For this review, take the finished solid that the model builds, in its own axes (mm). A direction names the side the tool comes from. Give positions to 0.01 mm unless a question says otherwise; leave off trailing zeros. Write each loop counter-clockwise with the first axis right and the second up, starting at its lowest first coordinate (ties: lowest second). Pieces come first, ordered by that corner, then holes.
Q1. For line 1 (Y direction, x = -1.5, z = 1.25); line 2 (Y direction, x = -20, z = 5); line 3 (Z direction, x = 0, y = 65.5) (1 decimal), list the stretches that pass through material, from the lowest coordinate up.
Q2. Insertion check: P1, Ø1, axis at x = 33.5, z = 5.5, coming from the +Y side; P2, Ø8, axis at x = -39.2, y = 39.2, coming from the +Z side; P3, Ø8, axis at x = 26, z = 13.5, coming from the -Y side. Each pin has a flat end and moves straight along its axis. Give the tip position at first contact, or say it passes through.
Q3. Mouldability with a two-part tool opening along X and no side actions: class faces 1 (the cylindrical face through (39.531, -36.668, 3.219)), 2 (the cylindrical face through (-14.77, -66.515, 6.574)), 3 (the flat face through (30, -55, 15.875)) as released by +X, released by -X, zero draft, split by the parting line, or undercut.
Q4. Machinability: for faces 4 (the cylindrical face through (36.668, 39.531, 3.219)), 5 (the flat face through (-28, -41, 6.35)), which of the approach directions +Z, -Z, +X, -X, +Y, -Y give a long, thin tool a straight path to every point of the face, cutting with its end or side? Answer none if there is none.
Q5. We need section A-A (z = 2). Write out the cut boundary in (x, y), then the cut area to 3 significant figures.
```python
from build123d import *

# Parameters (mm, degrees)
SKETCH1_R                      = 68.1355
SKETCH1_R_2                    = 49.0855
EXTRUDE1_DEPTH                 = 15.875
SKETCH2_R                      = 61.7855
EXTRUDE2_DEPTH                 = 9.525
TAP_DRILL_FOR_10_32_TAP1_D     = 4.0386
TAP_DRILL_FOR_10_32_TAP1_DEPTH = 12.7
TAP_DRILL_FOR_10_32_TAP1_TIP   = 1.213317848
CIRPATTERN1_COUNT              = 4
CIRPATTERN2_COUNT              = 4
CHAMFER1_SIZE                  = 2.54
CHAMFER1_SIZE2                 = 0.680590949


with BuildPart() as part:
    # Sketch1 → Extrude1 (new body)
    with BuildSketch(Plane.XY):
        Circle(SKETCH1_R)
        Circle(SKETCH1_R_2, mode=Mode.SUBTRACT)
    extrude(amount=EXTRUDE1_DEPTH)

    # Sketch2 → Extrude2 (cut)
    with BuildSketch(Plane.XY.offset(15.875)):
        Circle(SKETCH2_R)
    extrude(amount=-EXTRUDE2_DEPTH, mode=Mode.SUBTRACT)

    # Tap Drill for #10-32 Tap1
    with Locations(Plane(origin=(26.074327006, 62.948993887, 11.1125), x_dir=(-0.9238795325112864, 0.38268343236509067, 0), z_dir=(0.38268343236509067, 0.9238795325112864, 0))):
        with Locations((0, 0)):
            Hole(TAP_DRILL_FOR_10_32_TAP1_D / 2, depth=TAP_DRILL_FOR_10_32_TAP1_DEPTH)
            with Locations((0, 0, -(TAP_DRILL_FOR_10_32_TAP1_DEPTH + TAP_DRILL_FOR_10_32_TAP1_TIP / 2))):  # 118° drill point
                Cone(0, TAP_DRILL_FOR_10_32_TAP1_D / 2, TAP_DRILL_FOR_10_32_TAP1_TIP, mode=Mode.SUBTRACT)

    # Sketch4 → M3x0.5 Tapped Hole1 (revolve, cut)
    with BuildSketch(Plane(origin=(0, 68.1355, 11.1125), x_dir=(0, 0, 1), z_dir=(1, 0, 0))):
        Polygon((0, 0), (0, 9.387075774), (1.25, 8.636), (1.25, 0), align=None)
    m3x0_5_tapped_hole1 = revolve(axis=Axis((0, 74.4855, 11.1125), (0, -1, 0)), mode=Mode.SUBTRACT)

    # CirPattern1: M3x0.5 Tapped Hole1 ×4 about axis
    cirpattern1_axis = Axis((0, 0, 15.875), (0, 0, -1))
    for i in range(1, CIRPATTERN1_COUNT):
        add(m3x0_5_tapped_hole1.rotate(cirpattern1_axis, i * 360 / CIRPATTERN1_COUNT), mode=Mode.SUBTRACT)

    # Sketch8 → 1/4-20 Tapped Hole1 (revolve, cut)
    with BuildSketch(Plane(origin=(39.198817968, 39.198817968, 11.1125), x_dir=(0, -1, 0), z_dir=(1, 0, 0))):
        Polygon((0, 0), (0, 18.043816902), (2.5527, 16.51), (2.5527, 0), align=None)
    f_1_4_20_tapped_hole1 = revolve(axis=Axis((39.198817968, 39.198817968, 17.4625), (0, 0, -1)), mode=Mode.SUBTRACT)

    # CirPattern2: 1/4-20 Tapped Hole1 ×4 about axis
    cirpattern2_axis = Axis((0, 0, 0), (0, 0, 1))
    for i in range(1, CIRPATTERN2_COUNT):
        add(f_1_4_20_tapped_hole1.rotate(cirpattern2_axis, i * 360 / CIRPATTERN2_COUNT), mode=Mode.SUBTRACT)

    # Chamfer1
    chamfer1_edges = [part.edges().sort_by_distance(p)[0] for p in [
        (-68.1355, 0, 15.875),
    ]]
    chamfer1_side = [part.faces().sort_by_distance(p)[0] for p in [
        (-68.1355, 0, 7.9375),
    ]]
    chamfer(chamfer1_edges, length=CHAMFER1_SIZE, length2=CHAMFER1_SIZE2, reference=chamfer1_side[0])


solid = part.part
```
Computed:
1. line 1: y = -68.12 to -49.06, 49.06 to 68.12
1. line 2: y = -65.13 to -44.83, 44.83 to 65.13
1. line 3: z = 0 to 9.9, 12.4 to 15.9
2. P1: stops at y = 59.61
2. P2: stops at z = 6.35
2. P3: stops at y = -64.48
3. face 1: undercut
3. face 2: split by the parting line
3. face 3: zero draft
4. face 4: +Z, -Z
4. face 5: +Z
5. outline: circle Ø136.27 at (0, 0); hole circle Ø98.17 at (0, 0); hole circle Ø5.11 at (-39.2, -39.2); hole circle Ø5.11 at (-39.2, 39.2); hole circle Ø5.11 at (39.2, -39.2); hole circle Ø5.11 at (39.2, 39.2)
5. area: 6,930 mm2
